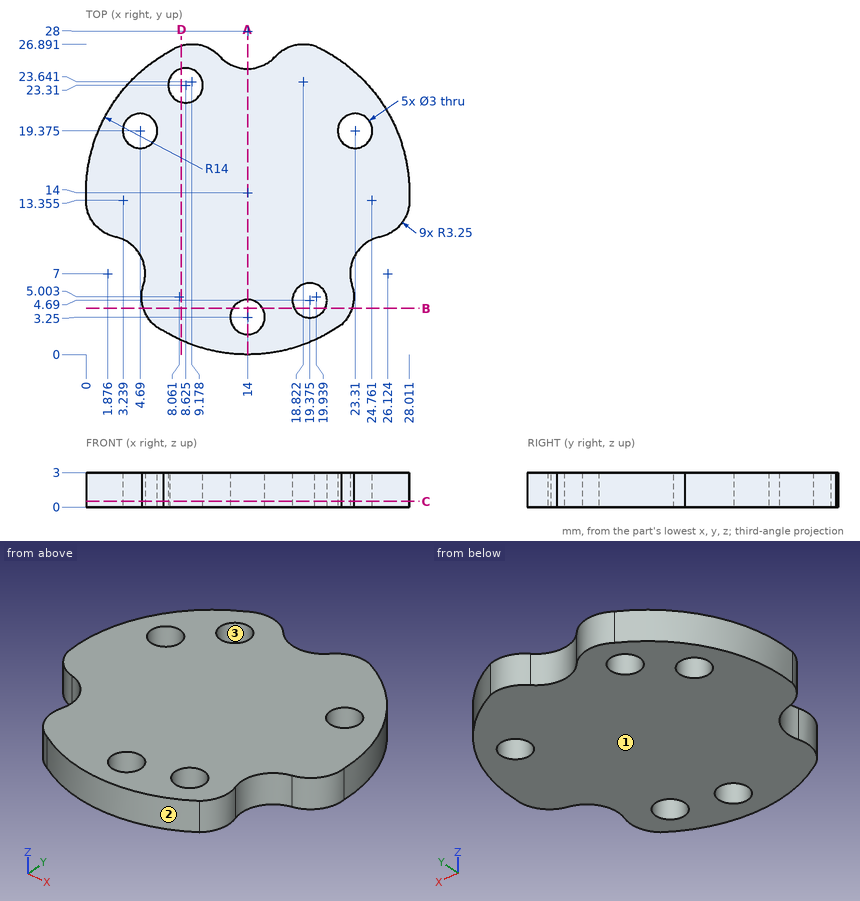
Study the drawing (mm; zero at the part's minimum x, y, z) and answer. Coordinates: 2 decimals unless noted, no trailing zeros. Write each loop counter-clockwise with the first axis right and the second up, starting at its lowest first coordinate (ties: lowest second). Pieces come first, ordered by that corner, then holes.
Q1. Determine the mould class of the marked faces 1, 2 and 3 for opening direction Y: released by +Y, released by -Y, zero draft, split by the parting line, or undercut.
Q2. Find the intervals of material crossed by line 1 (X direction, y = 19.5, z = 2.25) (1 decimal); line 2 (X direction, y = 4, z = 2.35); line 3 (Y direction, x = 19.25, z = 1.6) (1 decimal), in increasing order.
Q3. A cutting plane is placed at A-A, the plane x = 14. Give the vertices of the cut face in (y, z).
Q4. Each of these flat-tipped pins is pushed along its axis until it touches: pin 1 Ø2.5 at (x, y) = (4.69, 19.37) entering from -Z; pin 2 Ø4 at (x, y) = (8.63, 23.31) entering from +Z. Where does it stop, or does it pass through?
Q5. A cutting plane is placed at D-D, the plane x = 8.25. Give the vertices of the cut face in (y, z) (1 decimal).
Q6. A cutting plane is placed at C-C, the plane z = 0.5. State how many separate pieces and enclosed holes the cut face has, then the cut area to 3 significant figures.
Q7. A cutting plane is placed at B-B, the plane y = 4. Give the vertices of the cut face in (x, z), then the cut area to 3 significant figures.
Findings below:
1. face 1: zero draft
1. face 2: released by -Y
1. face 3: undercut
2. line 1: x = 1.1 to 3.2, 6.2 to 21.8, 24.8 to 26.9
2. line 2: x = 4.97 to 12.7, 15.3 to 18.04, 20.71 to 23.03
2. line 3: y = 1 to 3.2, 6.2 to 26.9
3. outline: (0, 0) - (1.75, 0) - (1.75, 3) - (0, 3) - close; (4.75, 0) - (24.75, 0) - (24.75, 3) - (4.75, 3) - close
4. pin 1: passes through
4. pin 2: stops at z = 3
5. outline: (1.2, 0) - (21.9, 0) - (21.9, 3) - (1.2, 3) - close; (24.8, 0) - (26.8, 0) - (26.8, 3) - (24.8, 3) - close
6. separate pieces: 1
6. enclosed holes: 5
6. area: 525 mm2
7. outline: (4.97, 0) - (12.7, 0) - (12.7, 3) - (4.97, 3) - close; (15.3, 0) - (18.04, 0) - (18.04, 3) - (15.3, 3) - close; (20.71, 0) - (23.03, 0) - (23.03, 3) - (20.71, 3) - close
7. area: 38.4 mm2
